```python
from build123d import *

# Parameters (mm, degrees)
F0_W     = 7.62
F0_H     = 7.62
F1_DEPTH = 3.175
F2_R     = 3.81
F3_DEPTH = 4.445
F4_R     = 1.905
F5_DEPTH = 4.445
F6_R     = 1.905
F7_DEPTH = 4.445


with BuildPart() as f1:
    # F0 (on Front) → F1 (new body, symmetric)
    with BuildSketch(Plane.XZ):
        with BuildLine():
            ThreePointArc((37.5221958358, -6.6102057198), (37.9552740824, -3.3177054311), (38.1, 0))
            ThreePointArc((38.1, 0), (37.9552740824, 3.3177054311), (37.5221958358, 6.6102057198))
            ThreePointArc((37.5221958358, 6.6102057198), (37.1447534541, 8.4780475837), (36.6743910775, 10.3246810652))
            ThreePointArc((36.6743910775, 10.3246810652), (34.3269138671, 16.5309704604), (30.9382695294, 22.2358601931))
            ThreePointArc((30.9382695294, 22.2358601931), (29.787779482, 23.7549614508), (28.5627733843, 25.2146381413))
            ThreePointArc((28.5627733843, 25.2146381413), (23.7549614508, 29.787779482), (18.2266395097, 33.4574298503))
            ThreePointArc((18.2266395097, 33.4574298503), (16.5309704604, 34.3269138671), (14.793948123, 35.1105268963))
            ThreePointArc((14.793948123, 35.1105268963), (8.4780475837, 37.1447534541), (1.905, 38.0523451971))
            ThreePointArc((1.905, 38.0523451971), (0, 38.1), (-1.905, 38.0523451971))
            ThreePointArc((-1.905, 38.0523451971), (-8.4780475837, 37.1447534541), (-14.793948123, 35.1105268963))
            ThreePointArc((-14.793948123, 35.1105268963), (-16.5309704604, 34.3269138671), (-18.2266395097, 33.4574298503))
            ThreePointArc((-18.2266395097, 33.4574298503), (-23.7549614508, 29.787779482), (-28.5627733843, 25.2146381413))
            ThreePointArc((-28.5627733843, 25.2146381413), (-29.787779482, 23.7549614508), (-30.9382695294, 22.2358601931))
            ThreePointArc((-30.9382695294, 22.2358601931), (-34.3269138671, 16.5309704604), (-36.6743910775, 10.3246810652))
            ThreePointArc((-36.6743910775, 10.3246810652), (-37.1447534541, 8.4780475837), (-37.5221958358, 6.6102057198))
            ThreePointArc((-37.5221958358, 6.6102057198), (-38.1, 0), (-37.5221958358, -6.6102057198))
            ThreePointArc((-37.5221958358, -6.6102057198), (-37.1447534541, -8.4780475837), (-36.6743910775, -10.3246810652))
            ThreePointArc((-36.6743910775, -10.3246810652), (-34.3269138671, -16.5309704604), (-30.9382695294, -22.2358601931))
            ThreePointArc((-30.9382695294, -22.2358601931), (-29.787779482, -23.7549614508), (-28.5627733843, -25.2146381413))
            ThreePointArc((-28.5627733843, -25.2146381413), (-23.7549614508, -29.787779482), (-18.2266395097, -33.4574298503))
            ThreePointArc((-18.2266395097, -33.4574298503), (-16.5309704604, -34.3269138671), (-14.793948123, -35.1105268963))
            ThreePointArc((-14.793948123, -35.1105268963), (-8.4780475837, -37.1447534541), (-1.905, -38.0523451971))
            ThreePointArc((-1.905, -38.0523451971), (0, -38.1), (1.905, -38.0523451971))
            ThreePointArc((1.905, -38.0523451971), (8.4780475837, -37.1447534541), (14.793948123, -35.1105268963))
            ThreePointArc((14.793948123, -35.1105268963), (16.5309704604, -34.3269138671), (18.2266395097, -33.4574298503))
            ThreePointArc((18.2266395097, -33.4574298503), (23.7549614508, -29.787779482), (28.5627733843, -25.2146381413))
            ThreePointArc((28.5627733843, -25.2146381413), (29.787779482, -23.7549614508), (30.9382695294, -22.2358601931))
            ThreePointArc((30.9382695294, -22.2358601931), (34.3269138671, -16.5309704604), (36.6743910775, -10.3246810652))
            ThreePointArc((36.6743910775, -10.3246810652), (37.1447534541, -8.4780475837), (37.5221958358, -6.6102057198))
        make_face()
        with BuildLine():
            ThreePointArc((31.5205710608, 3.81), (31.6925908627, 1.9084507878), (31.75, 0))
            ThreePointArc((31.75, 0), (31.6925908627, -1.9084507878), (31.5205710608, -3.81))
            ThreePointArc((31.5205710608, -3.81), (22.4506403027, -22.4506403027), (3.81, -31.5205710608))
            ThreePointArc((3.81, -31.5205710608), (0, -31.75), (-3.81, -31.5205710608))
            ThreePointArc((-3.81, -31.5205710608), (-22.4506403027, -22.4506403027), (-31.5205710608, -3.81))
            ThreePointArc((-31.5205710608, -3.81), (-31.75, 0), (-31.5205710608, 3.81))
            ThreePointArc((-31.5205710608, 3.81), (-22.4506403027, 22.4506403027), (-3.81, 31.5205710608))
            ThreePointArc((-3.81, 31.5205710608), (0, 31.75), (3.81, 31.5205710608))
            ThreePointArc((3.81, 31.5205710608), (22.4506403027, 22.4506403027), (31.5205710608, 3.81))
        make_face(mode=Mode.SUBTRACT)
        with BuildLine():
            ThreePointArc((36.6743910775, 10.3246810652), (37.1447534541, 8.4780475837), (37.5221958358, 6.6102057198))
            Line((37.5221958358, 6.6102057198), (43.7129880782, 8.0232136504))
            Line((43.7129880782, 8.0232136504), (42.8651833198, 11.7376889958))
            Line((42.8651833198, 11.7376889958), (36.6743910775, 10.3246810652))
        make_face()
        with BuildLine():
            Line((43.7129880782, -8.0232136504), (37.5221958358, -6.6102057198))
            ThreePointArc((37.5221958358, -6.6102057198), (37.1447534541, -8.4780475837), (36.6743910775, -10.3246810652))
            Line((36.6743910775, -10.3246810652), (42.8651833198, -11.7376889958))
            Line((42.8651833198, -11.7376889958), (43.7129880782, -8.0232136504))
        make_face()
        with BuildLine():
            ThreePointArc((28.5627733843, 25.2146381413), (29.787779482, 23.7549614508), (30.9382695294, 22.2358601931))
            Line((30.9382695294, 22.2358601931), (35.9028994431, 26.1950204349))
            Line((35.9028994431, 26.1950204349), (33.527403298, 29.1737983831))
            Line((33.527403298, 29.1737983831), (28.5627733843, 25.2146381413))
        make_face()
        with BuildLine():
            Line((35.9028994431, -26.1950204349), (30.9382695294, -22.2358601931))
            ThreePointArc((30.9382695294, -22.2358601931), (29.787779482, -23.7549614508), (28.5627733843, -25.2146381413))
            Line((28.5627733843, -25.2146381413), (33.527403298, -29.1737983831))
            Line((33.527403298, -29.1737983831), (35.9028994431, -26.1950204349))
        make_face()
        with BuildLine():
            ThreePointArc((14.793948123, 35.1105268963), (16.5309704604, 34.3269138671), (18.2266395097, 33.4574298503))
            Line((18.2266395097, 33.4574298503), (20.9818012531, 39.1785821614))
            Line((20.9818012531, 39.1785821614), (17.5491098664, 40.8316792075))
            Line((17.5491098664, 40.8316792075), (14.793948123, 35.1105268963))
        make_face()
        with BuildLine():
            Line((20.9818012531, -39.1785821614), (18.2266395097, -33.4574298503))
            ThreePointArc((18.2266395097, -33.4574298503), (16.5309704604, -34.3269138671), (14.793948123, -35.1105268963))
            Line((14.793948123, -35.1105268963), (17.5491098664, -40.8316792075))
            Line((17.5491098664, -40.8316792075), (20.9818012531, -39.1785821614))
        make_face()
        with BuildLine():
            ThreePointArc((-1.905, 38.0523451971), (0, 38.1), (1.905, 38.0523451971))
            Line((1.905, 38.0523451971), (1.905, 44.4023451971))
            Line((1.905, 44.4023451971), (-1.905, 44.4023451971))
            Line((-1.905, 44.4023451971), (-1.905, 38.0523451971))
        make_face()
        with BuildLine():
            Line((1.905, -44.4023451971), (1.905, -38.0523451971))
            ThreePointArc((1.905, -38.0523451971), (0, -38.1), (-1.905, -38.0523451971))
            Line((-1.905, -38.0523451971), (-1.905, -44.4023451971))
            Line((-1.905, -44.4023451971), (1.905, -44.4023451971))
        make_face()
        with BuildLine():
            ThreePointArc((-18.2266395097, 33.4574298503), (-16.5309704604, 34.3269138671), (-14.793948123, 35.1105268963))
            Line((-14.793948123, 35.1105268963), (-17.5491098664, 40.8316792075))
            Line((-17.5491098664, 40.8316792075), (-20.9818012531, 39.1785821614))
            Line((-20.9818012531, 39.1785821614), (-18.2266395097, 33.4574298503))
        make_face()
        with BuildLine():
            Line((-17.5491098664, -40.8316792075), (-14.793948123, -35.1105268963))
            ThreePointArc((-14.793948123, -35.1105268963), (-16.5309704604, -34.3269138671), (-18.2266395097, -33.4574298503))
            Line((-18.2266395097, -33.4574298503), (-20.9818012531, -39.1785821614))
            Line((-20.9818012531, -39.1785821614), (-17.5491098664, -40.8316792075))
        make_face()
        with BuildLine():
            ThreePointArc((-30.9382695294, 22.2358601931), (-29.787779482, 23.7549614508), (-28.5627733843, 25.2146381413))
            Line((-28.5627733843, 25.2146381413), (-33.527403298, 29.1737983831))
            Line((-33.527403298, 29.1737983831), (-35.9028994431, 26.1950204349))
            Line((-35.9028994431, 26.1950204349), (-30.9382695294, 22.2358601931))
        make_face()
        with BuildLine():
            Line((-33.527403298, -29.1737983831), (-28.5627733843, -25.2146381413))
            ThreePointArc((-28.5627733843, -25.2146381413), (-29.787779482, -23.7549614508), (-30.9382695294, -22.2358601931))
            Line((-30.9382695294, -22.2358601931), (-35.9028994431, -26.1950204349))
            Line((-35.9028994431, -26.1950204349), (-33.527403298, -29.1737983831))
        make_face()
        with BuildLine():
            ThreePointArc((-37.5221958358, 6.6102057198), (-37.1447534541, 8.4780475837), (-36.6743910775, 10.3246810652))
            Line((-36.6743910775, 10.3246810652), (-42.8651833198, 11.7376889958))
            Line((-42.8651833198, 11.7376889958), (-43.7129880782, 8.0232136504))
            Line((-43.7129880782, 8.0232136504), (-37.5221958358, 6.6102057198))
        make_face()
        with BuildLine():
            Line((-42.8651833198, -11.7376889958), (-36.6743910775, -10.3246810652))
            ThreePointArc((-36.6743910775, -10.3246810652), (-37.1447534541, -8.4780475837), (-37.5221958358, -6.6102057198))
            Line((-37.5221958358, -6.6102057198), (-43.7129880782, -8.0232136504))
            Line((-43.7129880782, -8.0232136504), (-42.8651833198, -11.7376889958))
        make_face()
        with BuildLine():
            ThreePointArc((31.5205710608, -3.81), (31.6925908627, -1.9084507878), (31.75, 0))
            ThreePointArc((31.75, 0), (31.6925908627, 1.9084507878), (31.5205710608, 3.81))
            Line((31.5205710608, 3.81), (3.81, 3.81))
            Line((3.81, 3.81), (3.81, -3.81))
            Line((3.81, -3.81), (31.5205710608, -3.81))
        make_face()
        with BuildLine():
            Line((3.81, 3.81), (3.81, 31.5205710608))
            ThreePointArc((3.81, 31.5205710608), (0, 31.75), (-3.81, 31.5205710608))
            Line((-3.81, 31.5205710608), (-3.81, 3.81))
            Line((-3.81, 3.81), (3.81, 3.81))
        make_face()
        Rectangle(F0_W, F0_H)
        with BuildLine():
            ThreePointArc((-3.81, -31.5205710608), (0, -31.75), (3.81, -31.5205710608))
            Line((3.81, -31.5205710608), (3.81, -3.81))
            Line((3.81, -3.81), (-3.81, -3.81))
            Line((-3.81, -3.81), (-3.81, -31.5205710608))
        make_face()
        with BuildLine():
            Line((-3.81, -3.81), (-3.81, 3.81))
            Line((-3.81, 3.81), (-31.5205710608, 3.81))
            ThreePointArc((-31.5205710608, 3.81), (-31.75, 0), (-31.5205710608, -3.81))
            Line((-31.5205710608, -3.81), (-3.81, -3.81))
        make_face()
    extrude(amount=F1_DEPTH, both=True)

    # F2 (on face) → F3 (join)
    with BuildSketch(Plane(origin=(0, 3.175, 0), x_dir=(-1, 0, 0), z_dir=(0, 1, 0))):
        with Locations((0, 34.29)):
            Circle(F2_R)
        with Locations((0, -34.29)):
            Circle(F2_R)
    extrude(amount=F3_DEPTH)

    # F4 (on face) → F5 (join)
    with BuildSketch(Plane(origin=(0, 7.62, 0), x_dir=(-1, 0, 0), z_dir=(0, 1, 0))):
        with Locations((0, 34.29)):
            Circle(F4_R)
    extrude(amount=F5_DEPTH)

    # F6 (on face) → F7 (cut)
    with BuildSketch(Plane(origin=(0, 7.62, 0), x_dir=(-1, 0, 0), z_dir=(0, 1, 0))):
        with Locations((0, -34.29)):
            Circle(F6_R)
    extrude(amount=-F7_DEPTH, mode=Mode.SUBTRACT)


solid = f1.part
```
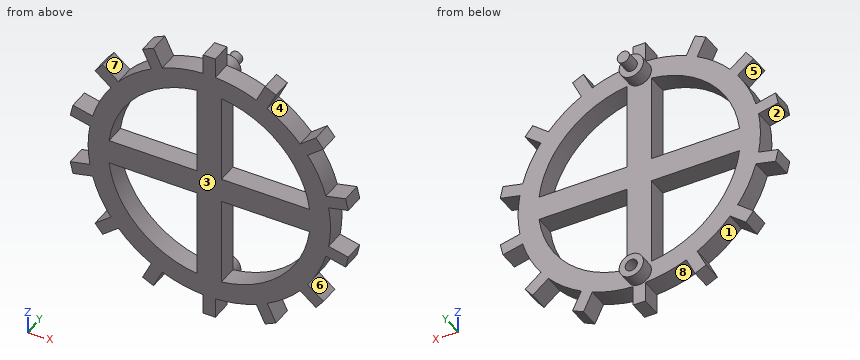
Geometry: final body of the model. Coordinates: model frame, mm. Face numbers are marked on the shaded views. A direction names the side the tool comes from. Round coordinates to 2 decimals unless told otherwise and drop trailing zeros. Order: outer loops, then holes, each group sorted by start corner. A loop starts at its lowest first (then second) coordinate and runs counter-clockwise, first axis right, second up. Notation, with made-up numbers: M -16.5,-6 L 11.5,-6 A22 ccw 11.5,1 Z; hole C 10.5,4 d3. An arc over 180 degrees is marked long. Use one line per item in the form item = value. Start each with the question number.
Q1. Material intervals for line 1 (Z direction, x = 0, y = 5.45) (3 decimals); line 2 (Z direction, x = 6, y = -1.5); line 3 (X direction, y = -0.5, z = -4), sorted ascending. Write a range as [from, to].
Q2. Cut plane B-B (y = 6). Return loops of the section in (x, z) (3 decimals), and give its area (3 significant figures).
Q3. Mould query, pull axis X, two halves, no side actions, for the marked faces 1, 2 and 3. Classes: +X half, -X half, draft (parallel to the pull), parting line (faces both ways), or undercut.
Q4. Cut plane C-C (x = 0). Return loops of the section in (y, z) (3 decimals), and give its area (3 significant figures).
Q5. Access query for the marked faces 4, 5, 6, 7 and 8. Directions: +Z, -Z, +X, -X, +Y, -Y. A direction counts if a zero-diameter tool reaches every point of the face in a straight line with its end or side. Return the directions, or none.
Q6. Cut plane A-A (x = 10). Return loops of the section in (y, z) (3 decimals).
Q7. Cut plane D-D (z = 20). Return loops of the section in (x, y) (3 decimals).
Q8. Pin query (flat end, axial travel): pin 1 Ø5 at (y, z) = (0, 41.5) entering from +X; pin 2 Ø6 at (y, z) = (5.5, 31) entering from +X; pin 3 Ø5 at (x, y) = (-16, -0.5) entering from +Z. Return the tip coordinate at first contact, or that it passes through.
Geometry results:
q1.line_1 = [-38.1, -36.195], [-32.385, -30.48], [30.48, 38.1]
q1.line_2 = [-37.62, -31.18], [-3.81, 3.81], [31.18, 37.62]
q1.line_3 = [-37.89, -31.5], [-3.81, 3.81], [31.5, 37.89]
q2.outline = C 0,-34.29 d7.62; C 0,34.29 d7.62; hole C 0,-34.29 d3.81
q2.area = 79.8 mm^2
q3.face_1 = undercut
q3.face_2 = -X half
q3.face_3 = draft
q4.outline = M -3.175,-44.402 L 3.175,-44.402 L 3.175,-38.1 L 7.62,-38.1 L 7.62,-36.195 L 3.175,-36.195 L 3.175,-32.385 L 7.62,-32.385 L 7.62,-30.48 L 3.175,-30.48 L 3.175,30.48 L 7.62,30.48 L 7.62,32.385 L 12.065,32.385 L 12.065,36.195 L 7.62,36.195 L 7.62,38.1 L 3.175,38.1 L 3.175,44.402 L -3.175,44.402 Z
q4.area = 632 mm^2
q5.face_4 = +Y, -Y
q5.face_5 = -X, +Y, -Y
q5.face_6 = +X, +Y, -Y
q5.face_7 = +Z, +Y, -Y
q5.face_8 = -Z, +Y, -Y
q6.outline = M -3.175,-36.764 L 3.175,-36.764 L 3.175,-30.134 L -3.175,-30.134 Z; M -3.175,-3.81 L 3.175,-3.81 L 3.175,3.81 L -3.175,3.81 Z; M -3.175,30.134 L 3.175,30.134 L 3.175,36.764 L -3.175,36.764 Z
q7.outline = M -32.429,-3.175 L -24.659,-3.175 L -24.659,3.175 L -32.429,3.175 Z; M -3.81,-3.175 L 3.81,-3.175 L 3.81,3.175 L -3.81,3.175 Z; M 24.659,-3.175 L 32.429,-3.175 L 32.429,3.175 L 24.659,3.175 Z
q8.pin_1 = 20.98
q8.pin_2 = 33.58
q8.pin_3 = 40.83
